from build123d import *

# Parameters (mm, degrees)
SKETCH1_R           = 4.28625
BOSS_EXTRUDE1_DEPTH = 50.8
FILLET2_R           = 2.54
SKETCH7_W           = 44.675933609
SKETCH7_H           = 44.675933609
CUT_EXTRUDE3_DEPTH  = 3.429
FILLET9_R           = 3.175
BOSS_EXTRUDE2_DEPTH = 30.1625
FILLET10_R          = 6.35


with BuildPart() as part:
    # Sketch1 → Boss-Extrude1 (new body)
    with BuildSketch(Plane(origin=(0, 0, 0), x_dir=(1, 0, 0), z_dir=(0, 1, 0))):
        with BuildLine():
            Line((13.462, 57.17106993), (-10.037787665, 10.037787665))
            Line((-10.037787665, 10.037787665), (-57.17106993, -13.462))
            Line((-57.17106993, -13.462), (-127, -13.462))
            Line((-127, -13.462), (-127, -18.542))
            Line((-127, -18.542), (0, -18.542))
            ThreePointArc((0, -18.542), (13.111173937, -13.111173937), (18.542, 0))
            Line((18.542, 0), (18.542, 127))
            Line((18.542, 127), (13.462, 127))
            Line((13.462, 127), (13.462, 57.17106993))
        make_face()
        with Locations(Location((0, 0, 0), (0, 0, 270))):
            Circle(SKETCH1_R, mode=Mode.SUBTRACT)
    extrude(amount=BOSS_EXTRUDE1_DEPTH)

    # Fillet2
    fillet2_edges = [part.edges().sort_by_distance(p)[0] for p in [
        (13.462, 25.4, -127),
        (18.542, 25.4, -127),
        (-127, 25.4, 13.462),
        (-127, 25.4, 18.542),
    ]]
    fillet(fillet2_edges, radius=FILLET2_R - 0.0001)  # a hair under: the kernel refuses the full size

    # Sketch7 → Cut-Extrude3 (cut)
    with BuildSketch(Plane(origin=(0, 50.8, 0), x_dir=(1, 0, 0), z_dir=(0, 1, 0))):
        with Locations((-17.511966805, 17.511966805)):
            Rectangle(SKETCH7_W, SKETCH7_H)
    extrude(amount=-CUT_EXTRUDE3_DEPTH, mode=Mode.SUBTRACT)

    # Fillet9
    fillet9_edges = [part.edges().sort_by_distance(p)[0] for p in [
        (4.826, 49.0855, -39.849933609),
        (4.826, 49.0855, 4.826),
        (-39.849933609, 49.0855, 4.826),
    ]]
    fillet(fillet9_edges, radius=FILLET9_R)

    # Sketch8 → Boss-Extrude2 (add, symmetric)
    with BuildSketch(Plane(origin=(0, 25.4, 0), x_dir=(1, 0, 0), z_dir=(0, 1, 0))):
        with BuildLine():
            Line((0, -13.462), (-124.46, -13.462))
            ThreePointArc((-124.46, -13.462), (-126.256051224, -14.205948776), (-127, -16.002))
            ThreePointArc((-127, -16.002), (-126.256051224, -17.798051224), (-124.46, -18.542))
            Line((-124.46, -18.542), (0, -18.542))
            ThreePointArc((0, -18.542), (13.111173937, -13.111173937), (18.542, 0))
            Line((18.542, 0), (18.542, 124.46))
            ThreePointArc((18.542, 124.46), (17.798051224, 126.256051224), (16.002, 127))
            ThreePointArc((16.002, 127), (14.205948776, 126.256051224), (13.462, 124.46))
            Line((13.462, 124.46), (13.462, 0))
            ThreePointArc((13.462, 0), (9.519071488, -9.519071488), (0, -13.462))
        make_face()
    extrude(amount=BOSS_EXTRUDE2_DEPTH, both=True)

    # Fillet10
    fillet10_edges = [part.edges().sort_by_distance(p)[0] for p in [
        (13.462, 25.4, -57.17106993),
        (-57.17106993, 25.4, 13.462),
        (-10.037787665, 23.6855, -10.037787665),
    ]]
    fillet(fillet10_edges, radius=FILLET10_R)


solid = part.part
Could you check a few things on this model? Use its own coordinates, in mm. A direction names the side the tool comes from. Give positions to 0.01 mm unless a question says otherwise; leave off trailing zeros. Order: outer loops, then holes, each group sorted by start corner. A loop starts at its lowest first (then second) coordinate and runs counter-clockwise, first axis right, second up.
1. I need wall thicknesses on L1, parallel to Y at x = 11, z = -25; L2, parallel to Z at x = -109.5, y = 29; L3, parallel to X at y = 50, z = -18.5. Which ranges of each line are inside material? Lowest first, please.
2. For faces 5 (the flat face through (4.826, 49, -18)), 6 (the flat face through (-22, 55.562, 16)), 7 (the cylindrical face through (9.623, -2.348, 9.414)), which set-ups out of +Z, -Z, +X, -X, +Y, -Y let a thin tool reach every point of the face, with its end or its side?
3. Suppose I cut it at C-C (z = -26.5). List the corners of the cut face in (x, y) for me, plus the area to 3 significant figures.
4. Will these pins go through, and if not, where does the flat tip stop? P1, Ø1, axis at y = 49, z = -11, coming from the -X side; P2, Ø2.5, axis at x = -26, y = 49.5, coming from the -Z side; P3, Ø12, axis at x = -9, y = 23.5, coming from the -Z side.
5. Suppose I cut it at B-B (x = -111.5). List the corners of the cut face in (y, z) for me.
6. We'd pull the mould along Z, two halves only. Please class faces 1 (the flat face through (-22, -4.763, 16)), 2 (the cylindrical face through (1.287, 23.354, 4.088)), 3 (the flat face through (-19, 49, 4.826)), 4 (the cylindrical face through (-127, 53, 16)): pulls with the +Z half, pulls with the -Z half, needs draft (parallel to the pull), parting line crosses it, or undercut.
Solved:
1. L1: y = 0 to 50.8
1. L2: z = 13.46 to 18.54
1. L3: x = 4.83 to 18.54
2. face 5: -Z, -X, +Y
2. face 6: +Z, -Z, +X, -X, +Y
2. face 7: -Z, -X, -Y
3. outline: (-1.83, 0) - (13.46, 0) - (13.46, -4.76) - (18.54, -4.76) - (18.54, 55.56) - (13.46, 55.56) - (13.46, 50.8) - (4.83, 50.8) - (4.83, 47.37) - (-1.83, 47.37) - close
3. area: 1,060 mm2
4. P1: stops at x = 4.83
4. P2: stops at z = 4.83
4. P3: stops at z = -24.15
5. outline: (-4.76, 13.46) - (55.56, 13.46) - (55.56, 18.54) - (-4.76, 18.54) - close
6. face 1: needs draft
6. face 2: undercut
6. face 3: pulls with the -Z half
6. face 4: parting line crosses it
